```python
from build123d import *

# Parameters (mm, degrees)
SKETCH2_R          = 1.778
CUT_EXTRUDE1_DEPTH = 8.777129933
SKETCH3_R          = 2.3241
CUT_EXTRUDE2_DEPTH = 3.048


with BuildPart() as part:
    # Sketch1 → Revolve3 (revolve)
    with BuildSketch(Plane(origin=(0, 0, 0), x_dir=(1, 0, 0), z_dir=(0, 1, 0))):
        with BuildLine():
            Line((0, 3.175), (0, -3.175))
            ThreePointArc((0, -3.175), (3.175, 0), (0, 3.175))
        make_face()
    revolve(axis=Axis((0, 0, -3.175), (0, 0, 1)))

    # Sketch2 → Cut-Extrude1 (cut, through all)
    with BuildSketch(Plane(origin=(3.175, 0, 0), x_dir=(0, 0, -1), z_dir=(1, 0, 0))):
        with Locations(Location((0, 0, 0), (0, 0, 180))):
            Circle(SKETCH2_R)
    extrude(amount=-CUT_EXTRUDE1_DEPTH, mode=Mode.SUBTRACT)

    # Sketch3 → Cut-Extrude2 (cut)
    with BuildSketch(Plane(origin=(3.175, 0, 0), x_dir=(0, 0, -1), z_dir=(1, 0, 0))):
        Circle(SKETCH3_R)
    extrude(amount=-CUT_EXTRUDE2_DEPTH, mode=Mode.SUBTRACT)


solid = part.part
```
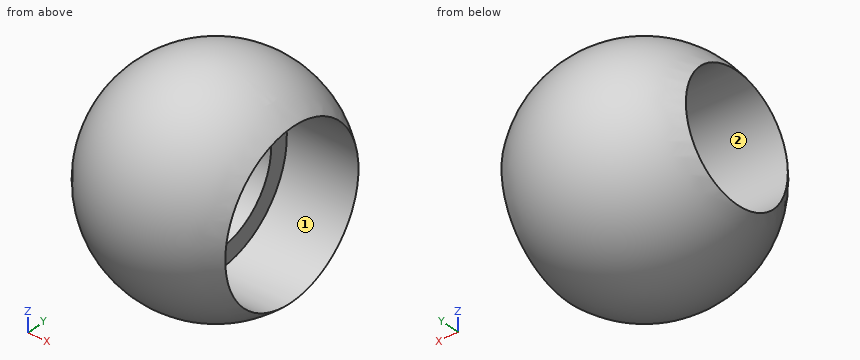
Can you work these out from the model? Positions are in its coordinate system, mm. Face numbers are marked on the shaded views. Round coordinates to 2 decimals unless told otherwise and drop trailing zeros. Loops run counter-clockwise (first coordinate to the right, second up) from the corner with the lowest first, then second, coordinate; pieces in that order, holes last. Notation, with made-up numbers: (-38, -13) -> (-26, -13) arc R21 ccw to (-26, 0) -> close; hole circle Ø6 at (60, 28.25). An arc over 180 degrees is marked (long way). One line per item, written item: value. Start each with the question number.
1. For pin 1 (1 mm diameter, centred on x = 0, y = -1.5, fed in from +Z), with a flat end and sliding along its axis, tell me the tip position at first contact or that it passes through.
2. If we section it at D-D, the plane y = 2.75: Write out the boundary of the cut face in (x, z), then the cut area to 3 significant figures.
3. If we mould it in two halves opening along Z, with no side actions, what happens to the marked faces 1 and 2? For each: pulls with the +Z half, pulls with the -Z half, needs draft (parallel to the pull), parting line crosses it, or undercut.
4. If I drill on probe 1 along Z at (x, y) = (0.7, 0.25); probe 2 along Z at (x, y) = (-0.85, -0.75); probe 3 along Y at (x, z) = (-2.4, -1.25), over which ranges is the centre line in solid material (lowest first)?
5. If we section it at A-A, the plane z = 0: Write out the boundary of the cut face in (x, y) (3 decimals).
6. If we section it at C-C, the plane x = -1.4: Write out the boundary of the cut face in (y, z), then the cut area to 3 significant figures.
Calculated:
1. pin 1: stops at z = 3.01
2. outline: circle Ø3.17 at (0, 0)
2. area: 7.91 mm²
3. face 1: undercut
3. face 2: undercut
4. probe 1: z = -3.09 to -2.31, 2.31 to 3.09
4. probe 2: z = -2.97 to -1.61, 1.61 to 2.97
4. probe 3: y = -1.66 to -1.26, 1.26 to 1.66
5. outline: (-2.63, -1.778) arc R3.175 ccw to (2.163, -2.324) -> (0.127, -2.324) -> (0.127, -1.778) -> close; (-2.63, 1.778) -> (0.127, 1.778) -> (0.127, 2.324) -> (2.163, 2.324) arc R3.175 ccw to start
6. outline: circle Ø5.7 at (0, 0); hole circle Ø3.56 at (0, 0)
6. area: 15.6 mm²
